from build123d import *
from build123d.topology import SkipClean

# Parameters (mm, degrees)
SKETCH1_R           = 10
BOSS_EXTRUDE1_DEPTH = 50
SKETCH2_R           = 10
BOSS_EXTRUDE2_DEPTH = 50
BOSS_EXTRUDE3_START = 30
SKETCH4_R           = 10
BOSS_EXTRUDE3_DEPTH = 70


with BuildPart() as part:
    # Sketch1 → Boss-Extrude1 (new body)
    with BuildSketch(Plane.XY):
        Circle(SKETCH1_R)
    extrude(amount=BOSS_EXTRUDE1_DEPTH)

    # Sketch2 → Boss-Extrude2 (add)
    with SkipClean():  # the faces are left unmerged after this step: merging them gives an invalid solid
        with BuildSketch(Plane(origin=(0, 0, 0), x_dir=(1, 0, 0), z_dir=(0, 1, 0))):
            with Locations(Location((0, -40, 0), (0, 0, 270))):
                Circle(SKETCH2_R)
        extrude(amount=BOSS_EXTRUDE2_DEPTH)

    # Sketch4 → Boss-Extrude3 (add)
    with SkipClean():  # the faces are left unmerged after this step: merging them gives an invalid solid
        with BuildSketch(Plane.XY.offset(BOSS_EXTRUDE3_START)):
            with Locations((0, 40)):
                Circle(SKETCH4_R)
        extrude(amount=BOSS_EXTRUDE3_DEPTH)


solid = part.part
Verification items for the finished model (mm, model axes). A direction names the side the tool comes from. Give positions to 0.01 mm unless a question says otherwise; leave off trailing zeros. Write each loop counter-clockwise with the first axis right and the second up, starting at its lowest first coordinate (ties: lowest second). Pieces come first, ordered by that corner, then holes. Notation, with made-up numbers: M -11,67 L -1,67 A10 ccw -1,74 Z; hole C 30.5,19.25 d11. An arc over 180 degrees is marked long. Put each result on its own line as item: value. Start each with the question number.
1. Draft check along Y on faces 1 (the face through (0, 50, 40)), 2 (the face through (10, 40, 33)), 3 (the face through (0, 40, 30)). Enter one of: +Y half, -Y half, draft (parallel to the pull), parting line (faces both ways), or undercut.
2. Section check A-A (y = 24.5). Record the cut outline in (x, z).
3. Section check D-D (x = -4.75). Record the cut outline in (y, z).
4. Set-up check for faces 4 (the face through (-10, 46, 40)), 5 (the face through (-10, 40, 76)), 6 (the face through (0, 0, 50)), 7 (the face through (8.43, 19.72, 45.38)): record each of +Z, -Z, +X, -X, +Y, -Y from which the full face is reachable in a straight line by a thin tool's end or side.
5. Section check B-B (x = 3). Record the cut outline in (y, z), and give its area (3 significant figures).
6. Scan lines: line 1 along Z through (x, y) = (-2, 44); line 2 along Y through (x, z) = (0.5, 81); line 3 along Y through (x, z) = (0.25, 41). Record each from-to range of solid material in increasing order. Write a range as [from, to].
7. Go/stop test with flat-tipped pins: pin 1 Ø5 at (y, z) = (-4, 47.5) entering from -X; pin 2 Ø5 at (y, z) = (24.5, 46) entering from -X; pin 3 Ø12 at (y, z) = (31.5, 61.5) entering from +X; pin 4 Ø10 at (y, z) = (-1.5, 48.5) entering from +X. Record where each tip stops, or that it passes through.
Answer list:
1. face 1: +Y half
1. face 2: undercut
1. face 3: draft
2. outline: C 0,40 d20
3. outline: M -8.8,0 L 8.8,0 L 8.8,31.2 L 31.2,31.2 L 31.2,30 L 48.8,30 L 48.8,31.2 L 50,31.2 L 50,48.8 L 48.8,48.8 L 48.8,100 L 31.2,100 L 31.2,48.8 L 8.8,48.8 L 8.8,50 L -8.8,50 Z
4. face 4: -X, +Y
4. face 5: +Z
4. face 6: +Z, +X, -X, -Y
4. face 7: none
5. outline: M -9.54,0 L 9.54,0 L 9.54,30.46 L 30.46,30.46 L 30.46,30 L 49.54,30 L 49.54,30.46 L 50,30.46 L 50,49.54 L 49.54,49.54 L 49.54,100 L 30.46,100 L 30.46,49.54 L 9.54,49.54 L 9.54,50 L -9.54,50 Z
5. area: 2,700 mm2
6. line 1: [30, 100]
6. line 2: [30.01, 49.99]
6. line 3: [-10, 50]
7. pin 1: x = -9.89
7. pin 2: x = -9.37
7. pin 3: x = 9.68
7. pin 4: x = 10
